Geometry check sheet. Reference: the model listing, model coordinates, mm. A direction names the side the tool comes from. Coordinates: 2 decimals unless noted, no trailing zeros. Loops run counter-clockwise (first coordinate to the right, second up) from the corner with the lowest first, then second, coordinate; pieces in that order, holes last. Notation, with made-up numbers: M -35,41.25 L -28,41.25 A24 ccw -28,67.25 Z; hole C 6,75.25 d5. An arc over 180 degrees is marked long. One line per question, with ' | ' between items. Start each with the question number.
from build123d import *

# Parameters (mm, degrees)
EXTRUDE_THIN1_DEPTH = 80
BOSS_EXTRUDE1_DEPTH = 10
SKETCH2_3_R         = 20
BOSS_EXTRUDE2_DEPTH = 25
CUT_EXTRUDE1_REACH  = 158.605
SKETCH3_3_R         = 10
SKETCH3_3_W         = 5
SKETCH3_3_H         = 10.317541634
CUT_EXTRUDE2_DEPTH  = 10
HOLE1_D             = 40
HOLE1_DEPTH         = 10
SKETCH6_R           = 25
BOSS_EXTRUDE3_DEPTH = 10
RIB17_START         = -5
RIB17_DEPTH         = 10
RIB18_START         = -5
RIB18_DEPTH         = 10
RIB26_START         = -5
RIB26_DEPTH         = 10
HOLE2_D             = 30
HOLE3_D             = 20
HOLE3_DEPTH         = 10


with BuildPart() as part:
    # Sketch1 → Extrude-Thin1 (new body)
    with BuildSketch(Plane(origin=(0, 0, 0), x_dir=(0, 0, -1), z_dir=(1, 0, 0))):
        Polygon((0, 0), (-60, 0), (-60, 80), (-10, 80), (-10, 70), (-50, 70), (-50, 10), (0, 10), align=None)
    extrude(amount=-EXTRUDE_THIN1_DEPTH)

    # Sketch2 → Boss-Extrude1 (add)
    with BuildSketch(Plane(origin=(0, 0, 10), x_dir=(-1, 0, 0), z_dir=(0, 0, -1))):
        with BuildLine():
            Line((40, 80), (80, 80))
            Line((80, 80), (57.398181668, 119.864242224))
            ThreePointArc((57.398181668, 119.864242224), (59.338609482, 115.100802223), (60, 110))
            ThreePointArc((60, 110), (54.142135624, 95.857864376), (40, 90))
            Line((40, 90), (40, 80))
        make_face()
        with BuildLine():
            Line((0, 80), (40, 80))
            Line((40, 80), (40, 90))
            ThreePointArc((40, 90), (22.718726255, 99.932349938), (22.601818332, 119.864242224))
            Line((22.601818332, 119.864242224), (0, 80))
        make_face()
    extrude(amount=-BOSS_EXTRUDE1_DEPTH)

    # Sketch2<3> → Boss-Extrude2 (add)
    with BuildSketch(Plane(origin=(0, 0, 10), x_dir=(-1, 0, 0), z_dir=(0, 0, -1))):
        with Locations((40, 110)):
            Circle(SKETCH2_3_R)
    extrude(amount=-BOSS_EXTRUDE2_DEPTH)

    # Sketch3 → Cut-Extrude1 (cut, up to next)
    with BuildSketch(Plane.XY.offset(35), mode=Mode.PRIVATE) as cut_extrude1_sk1:
        with BuildLine():
            ThreePointArc((-37.5, 119.682458366), (-40, 120), (-42.5, 119.682458366))
            Line((-42.5, 119.682458366), (-37.5, 119.682458366))
        make_face()
    cut_extrude1_tool1 = extrude(cut_extrude1_sk1.sketch, amount=-CUT_EXTRUDE1_REACH, mode=Mode.PRIVATE) & part.part
    # Sketch3 → Cut-Extrude1 (cut, up to next)
    with BuildSketch(Plane.XY.offset(35), mode=Mode.PRIVATE) as cut_extrude1_sk2:
        with BuildLine():
            Line((-37.5, 119.682458366), (-42.5, 119.682458366))
            ThreePointArc((-42.5, 119.682458366), (-46.123724357, 102.09430585), (-30, 110))
            ThreePointArc((-30, 110), (-32.09430585, 116.123724357), (-37.5, 119.682458366))
        make_face()
    cut_extrude1_tool2 = extrude(cut_extrude1_sk2.sketch, amount=-CUT_EXTRUDE1_REACH, mode=Mode.PRIVATE) & part.part
    add(cut_extrude1_tool1.solids().sort_by_distance((-40, 119.809649, 35))[0], mode=Mode.SUBTRACT)
    add(cut_extrude1_tool2.solids().sort_by_distance((-40, 109.96673, 35))[0], mode=Mode.SUBTRACT)

    # Sketch3<3> → Cut-Extrude2 (cut)
    with BuildSketch(Plane.XY.offset(35)):
        with Locations((-40, 110)):
            Circle(SKETCH3_3_R)
        with Locations((-40, 124.841229183)):
            Rectangle(SKETCH3_3_W, SKETCH3_3_H)
    extrude(amount=-CUT_EXTRUDE2_DEPTH, mode=Mode.SUBTRACT)

    # Hole1
    with Locations(Plane(origin=(0, 10, 0), x_dir=(1, 0, 0), z_dir=(0, 1, 0))):
        with Locations((-40, 0)):
            Hole(HOLE1_D / 2, depth=HOLE1_DEPTH)

    # Sketch6 → Boss-Extrude3 (add)
    with BuildSketch(Plane.XY.offset(60)):
        with Locations((-40, 40)):
            Circle(SKETCH6_R)
    extrude(amount=BOSS_EXTRUDE3_DEPTH)

    # Rib17: read off the stored shape, not the designer's step
    # Rib17 outline → Rib17 (add)
    with BuildSketch(Plane(origin=(0, 40, 0), x_dir=(-1, 0, 0), z_dir=(0, -1, 0)).offset(RIB17_START)):
        Polygon((15.505102572, -70), (15.505102572, -60), (0, -60), (15, -70), align=None)
    extrude(amount=RIB17_DEPTH)

    # Rib18: read off the stored shape, not the designer's step
    # Rib18 outline → Rib18 (add)
    with BuildSketch(Plane(origin=(0, 40, 0), x_dir=(-1, 0, 0), z_dir=(0, -1, 0)).offset(RIB18_START)):
        Polygon((80, -60), (64.494897428, -60), (64.494897428, -70), (65, -70), align=None)
    extrude(amount=RIB18_DEPTH)

    # Rib26: read off the stored shape, not the designer's step
    # Rib26 outline → Rib26 (add)
    with BuildSketch(Plane(origin=(-40, 0, 0), x_dir=(0, 0, -1), z_dir=(1, 0, 0)).offset(RIB26_START)):
        with BuildLine():
            Line((-70, 80), (-70, 64.494897428))
            Line((-70, 64.494897428), (-60, 64.494897428))
            Line((-60, 64.494897428), (-60, 80))
            Line((-60, 80), (-20, 80))
            Line((-20, 80), (-20, 90.635083269))
            Line((-20, 90.635083269), (-35, 90.635083269))
            Line((-35, 90.635083269), (-35, 90))
            Line((-35, 90), (-60, 90))
            ThreePointArc((-60, 90), (-67.071067812, 87.071067812), (-70, 80))
        make_face()
    extrude(amount=RIB26_DEPTH)

    # Hole2 (through all)
    with Locations(Plane.XY.offset(70)):
        with Locations((-40, 40)):
            Hole(HOLE2_D / 2)

    # Hole3
    with Locations(Plane(origin=(0, 80, 0), x_dir=(1, 0, 0), z_dir=(0, 1, 0))):
        with Locations((-20, -35)):
            hole3 = Hole(HOLE3_D / 2, depth=HOLE3_DEPTH)

    # Mirror1: Hole3 across plane
    add(hole3.mirror(Plane(origin=(-40, 0, 0), x_dir=(0, 0, 1), z_dir=(1, 0, 0))), mode=Mode.SUBTRACT)


solid = part.part
1. Sectioned sample at B-B (x = -40). Record the cut outline in (y, z), and give its area (3 significant figures).
2. Depth check by flat-ended pin: pin 1 Ø10.5 at (x, y) = (-20.5, 107.5) entering from +Z; pin 2 Ø5 at (x, z) = (-41, 50) entering from +Y; pin 3 Ø8 at (y, z) = (125.5, 30.5) entering from +X. Enter the tip coordinate at first touch or a pass-through.
3. Draft check along X on faces 1 (the cylindrical face through (-57.533, 57.822, 64.93)), 2 (the flat face through (-66, 66, 60)), 3 (the cylindrical face through (-24.614, 74.93, 43.872)). Enter one of: +X half, -X half, draft (parallel to the pull), parting line (faces both ways), or undercut.
4. Sectioned sample at A-A (y = 40). Record the cut outline in (x, z).
5. Sectioned sample at D-D (x = -17.5). Record the cut outline in (y, z).
6. Sectioned sample at C-C (z = 11.5). Record the cut outline in (x, y).
7. Tool access check on faces 4 (the flat face through (-39, 10, 31)), 5 (the flat face through (-70, 35, 64)), 6 (the flat face through (-39, 13, 60)), 7 (the flat face through (-39, 94, 10)). Record the directions out of +Z, -Z, +X, -X, +Y, -Y that give a thin tool (end or side, any length) a straight path to the whole face; none if there is none.
8. Thickness scan on line 1 (X direction, y = 73, z = 35); line 2 (Y direction, x = -47, z = 35.5); line 3 (Z direction, x = -60, y = 75). Record the ranges inside material, lowest first.
Result:
1) outline: M 0,20 L 10,20 L 10,50 L 25,50 L 25,70 L 15,70 L 15,60 L 0,60 Z; M 55,50 L 70,50 L 70,10 L 100,10 L 100,35 L 90,35 L 90,60 A10 ccw 80,70 L 55,70 Z; M 120,10 L 130,10 L 130,25 L 120,25 Z | area: 2,530 mm2
2) pin 1: stops at z = 35 | pin 2: stops at y = 90 | pin 3: stops at x = -23.64
3) face 1: -X half | face 2: draft | face 3: undercut
4) outline: M -80,50 L -55,50 L -55,70 L -65,70 L -80,60 Z; M -25,50 L 0,50 L 0,60 L -15,70 L -25,70 Z
5) outline: M 0,0 L 10,0 L 10,50 L 70,50 L 70,44.68 L 80,44.68 L 80,60 L 50.9,60 L 50.9,70 L 29.1,70 L 29.1,60 L 0,60 Z; M 70,10 L 110.87,10 L 110.87,20 L 80,20 L 80,25.32 L 70,25.32 Z
6) outline: M -80,0 L -56.36,0 L -56.36,10 L -80,10 Z; M -80,70 L 0,70 L 0,80 L -22.6,119.86 A20 ccw -57.4,119.86 L -80,80 Z; M -23.64,0 L 0,0 L 0,10 L -23.64,10 Z; hole C -40,110 d20
7) face 4: -Z, +X, -X | face 5: +Z, -X, -Y | face 6: +Z, -Y | face 7: -Z, +X, -X, +Y
8) line 1: x = -80 to -70, -50 to -30, -10 to 0 | line 2: y = 0 to 10, 70 to 80 | line 3: z = 10 to 25, 45 to 60
